Verification items for the finished model (mm, model axes). A direction names the side the tool comes from. Round coordinates to 2 decimals unless told otherwise and drop trailing zeros. Write each loop counter-clockwise with the first axis right and the second up, starting at its lowest first coordinate (ties: lowest second). Pieces come first, ordered by that corner, then holes. Notation, with made-up numbers: (-20, 31.5) -> (-12, 31.5) arc R17 cw to (-12, 60.5) -> close; hole circle Ø9 at (63, -10). An arc over 180 degrees is marked (long way). Answer as a JSON object with one key per item and string values. Group by question number.
(1) Draft check along Y on faces 1 (the face through (3.75, 1, 0)), 2 (the face through (1.85, 41.17, -4.13)). Enter one of: released by +Y, released by -Y, zero draft, split by the parting line, or undercut.
(2) Sectioned sample at C-C on y = -21.5. Record the cut outline in (x, z).
(3) Gauge pin test, flat ends, axial feed: pin 1 Ø4.5 at (y, z) = (46.895, 19.26) entering from +X; pin 2 Ø3 at (y, z) = (-7.075, 11.55) entering from +X. Record the tip position at first contact, or that the pin passes through.
(4) Sectioned sample at A-A on y = 4. Record the cut outline in (x, z) (3 decimals), and give its area (3 significant figures).
(5) Set-up check for faces 3 (the face through (1.85, 30.26, 17.67)), 4 (the face through (1.23, 5.01, -24.08)): record each of +Z, -Z, +X, -X, +Y, -Y from which the full face is reachable in a straight line by a thin tool's end or side.
(6) Sectioned sample at B-B on z = -19.29. Count the separate pieces of the cut face and the enclosed holes in it, and give its area (3 significant figures).
```python
from build123d import *

# Parameters (mm, degrees)
SKETCH1_W           = 50
SKETCH1_H           = 100
BOSS_EXTRUDE1_DEPTH = 3.75
SKETCH2_R           = 2
CUT_EXTRUDE1_DEPTH  = 3.75
SKETCH5_R           = 1.2
CUT_EXTRUDE2_DEPTH  = 1.875


with BuildPart() as part:
    # Sketch1 → Boss-Extrude1 (new body)
    with BuildSketch(Plane(origin=(0, 0, 0), x_dir=(0, 0, -1), z_dir=(1, 0, 0))):
        Rectangle(SKETCH1_W, SKETCH1_H)
    extrude(amount=BOSS_EXTRUDE1_DEPTH)

    # Sketch2 → Cut-Extrude1 (cut)
    with BuildSketch(Plane.ZY):
        with Locations((-19.29, 46.895)):
            Circle(SKETCH2_R)
        with Locations((-11.58, 46.895)):
            Circle(SKETCH2_R)
        with Locations((-3.87, 46.895)):
            Circle(SKETCH2_R)
        with Locations((3.84, 46.895)):
            Circle(SKETCH2_R)
        with Locations((11.55, 46.895)):
            Circle(SKETCH2_R)
        with Locations((19.26, 46.895)):
            Circle(SKETCH2_R)
        with Locations((-19.29, 39.185)):
            Circle(SKETCH2_R)
        with Locations((-11.58, 39.185)):
            Circle(SKETCH2_R)
        with Locations((-3.87, 39.185)):
            Circle(SKETCH2_R)
        with Locations((3.84, 39.185)):
            Circle(SKETCH2_R)
        with Locations((11.55, 39.185)):
            Circle(SKETCH2_R)
        with Locations((19.26, 39.185)):
            Circle(SKETCH2_R)
        with Locations((-19.29, 31.475)):
            Circle(SKETCH2_R)
        with Locations((-11.58, 31.475)):
            Circle(SKETCH2_R)
        with Locations((-3.87, 31.475)):
            Circle(SKETCH2_R)
        with Locations((3.84, 31.475)):
            Circle(SKETCH2_R)
        with Locations((11.55, 31.475)):
            Circle(SKETCH2_R)
        with Locations((19.26, 31.475)):
            Circle(SKETCH2_R)
        with Locations((-19.29, 23.765)):
            Circle(SKETCH2_R)
        with Locations((-11.58, 23.765)):
            Circle(SKETCH2_R)
        with Locations((-3.87, 23.765)):
            Circle(SKETCH2_R)
        with Locations((3.84, 23.765)):
            Circle(SKETCH2_R)
        with Locations((11.55, 23.765)):
            Circle(SKETCH2_R)
        with Locations((19.26, 23.765)):
            Circle(SKETCH2_R)
        with Locations((-19.29, 16.055)):
            Circle(SKETCH2_R)
        with Locations((-11.58, 16.055)):
            Circle(SKETCH2_R)
        with Locations((-3.87, 16.055)):
            Circle(SKETCH2_R)
        with Locations((3.84, 16.055)):
            Circle(SKETCH2_R)
        with Locations((11.55, 16.055)):
            Circle(SKETCH2_R)
        with Locations((19.26, 16.055)):
            Circle(SKETCH2_R)
        with Locations((-19.29, 8.345)):
            Circle(SKETCH2_R)
        with Locations((-11.58, 8.345)):
            Circle(SKETCH2_R)
        with Locations((-3.87, 8.345)):
            Circle(SKETCH2_R)
        with Locations((3.84, 8.345)):
            Circle(SKETCH2_R)
        with Locations((11.55, 8.345)):
            Circle(SKETCH2_R)
        with Locations((19.26, 8.345)):
            Circle(SKETCH2_R)
        with Locations((-19.29, 0.635)):
            Circle(SKETCH2_R)
        with Locations((-11.58, 0.635)):
            Circle(SKETCH2_R)
        with Locations((-3.87, 0.635)):
            Circle(SKETCH2_R)
        with Locations((3.84, 0.635)):
            Circle(SKETCH2_R)
        with Locations((11.55, 0.635)):
            Circle(SKETCH2_R)
        with Locations((19.26, 0.635)):
            Circle(SKETCH2_R)
        with Locations((-19.29, -7.075)):
            Circle(SKETCH2_R)
        with Locations((-11.58, -7.075)):
            Circle(SKETCH2_R)
        with Locations((-3.87, -7.075)):
            Circle(SKETCH2_R)
        with Locations((3.84, -7.075)):
            Circle(SKETCH2_R)
        with Locations((11.55, -7.075)):
            Circle(SKETCH2_R)
        with Locations((19.26, -7.075)):
            Circle(SKETCH2_R)
        with Locations((-19.29, -14.785)):
            Circle(SKETCH2_R)
        with Locations((-11.58, -14.785)):
            Circle(SKETCH2_R)
        with Locations((-3.87, -14.785)):
            Circle(SKETCH2_R)
        with Locations((3.84, -14.785)):
            Circle(SKETCH2_R)
        with Locations((11.55, -14.785)):
            Circle(SKETCH2_R)
        with Locations((19.26, -14.785)):
            Circle(SKETCH2_R)
        with Locations((-19.29, -22.495)):
            Circle(SKETCH2_R)
        with Locations((-11.58, -22.495)):
            Circle(SKETCH2_R)
        with Locations((-3.87, -22.495)):
            Circle(SKETCH2_R)
        with Locations((3.84, -22.495)):
            Circle(SKETCH2_R)
        with Locations((11.55, -22.495)):
            Circle(SKETCH2_R)
        with Locations((19.26, -22.495)):
            Circle(SKETCH2_R)
        with Locations((-19.29, -30.205)):
            Circle(SKETCH2_R)
        with Locations((-11.58, -30.205)):
            Circle(SKETCH2_R)
        with Locations((-3.87, -30.205)):
            Circle(SKETCH2_R)
        with Locations((3.84, -30.205)):
            Circle(SKETCH2_R)
        with Locations((11.55, -30.205)):
            Circle(SKETCH2_R)
        with Locations((19.26, -30.205)):
            Circle(SKETCH2_R)
        with Locations((-19.29, -37.915)):
            Circle(SKETCH2_R)
        with Locations((-11.58, -37.915)):
            Circle(SKETCH2_R)
        with Locations((-3.87, -37.915)):
            Circle(SKETCH2_R)
        with Locations((3.84, -37.915)):
            Circle(SKETCH2_R)
        with Locations((11.55, -37.915)):
            Circle(SKETCH2_R)
        with Locations((19.26, -37.915)):
            Circle(SKETCH2_R)
        with Locations((-19.29, -45.625)):
            Circle(SKETCH2_R)
        with Locations((-11.58, -45.625)):
            Circle(SKETCH2_R)
        with Locations((-3.87, -45.625)):
            Circle(SKETCH2_R)
        with Locations((3.84, -45.625)):
            Circle(SKETCH2_R)
        with Locations((11.55, -45.625)):
            Circle(SKETCH2_R)
        with Locations((19.26, -45.625)):
            Circle(SKETCH2_R)
    extrude(amount=-CUT_EXTRUDE1_DEPTH, mode=Mode.SUBTRACT)

    # Sketch5 → Cut-Extrude2 (cut)
    with BuildSketch(Plane(origin=(0, 0, -25), x_dir=(-1, 0, 0), z_dir=(0, 0, -1))):
        with Locations((-1.875, 4)):
            Circle(SKETCH5_R)
        with Locations((-1.875, -45)):
            Circle(SKETCH5_R)
    extrude(amount=-CUT_EXTRUDE2_DEPTH, mode=Mode.SUBTRACT)


solid = part.part
```
Computed values:
{
 "1": {"face 1": "zero draft", "face 2": "undercut"},
 "2": {"outline": "(0, -25) -> (3.75, -25) -> (3.75, -21.02) -> (0, -21.02) -> close; (0, -17.56) -> (3.75, -17.56) -> (3.75, -13.31) -> (0, -13.31) -> close; (0, -9.85) -> (3.75, -9.85) -> (3.75, -5.6) -> (0, -5.6) -> close; (0, -2.14) -> (3.75, -2.14) -> (3.75, 2.11) -> (0, 2.11) -> close; (0, 5.57) -> (3.75, 5.57) -> (3.75, 9.82) -> (0, 9.82) -> close; (0, 13.28) -> (3.75, 13.28) -> (3.75, 17.53) -> (0, 17.53) -> close; (0, 20.99) -> (3.75, 20.99) -> (3.75, 25) -> (0, 25) -> close"},
 "3": {"pin 1": "x = 3.75", "pin 2": "through"},
 "4": {"outline": "(0, -25) -> (0.675, -25) -> (0.675, -23.125) -> (3.075, -23.125) -> (3.075, -25) -> (3.75, -25) -> (3.75, 25) -> (0, 25) -> close", "area": "183 mm2"},
 "5": {"face 3": "+X, -X", "face 4": "-Z"},
 "6": {"separate pieces": "14", "enclosed holes": "0", "area": "180 mm2"}
}
